Check sheet for the drawn part. Datum: minimum x, y, z corner. Units: mm. A direction names the side the tool comes from. Coordinates: 2 decimals unless noted, no trailing zeros. Order: outer loops, then holes, each group sorted by start corner. A loop starts at its lowest first (then second) coordinate and runs counter-clockwise, first axis right, second up. Notation, with made-up numbers: (-1.5, 58) - (35.5, 58) arc R22 cw to (35.5, 95) - close; hole circle Ø1 at (47, 48). An arc over 180 degrees is marked (long way). One line per item, written item: value. Start each with the question number.
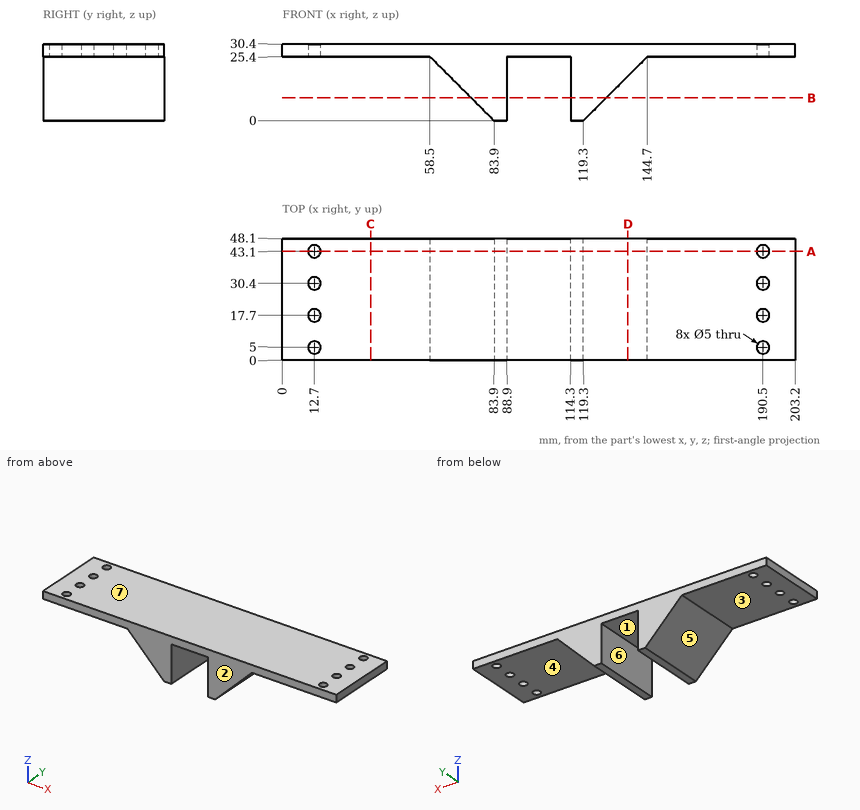
Q1. Material ranges on probe 1 along Y at (x, z) = (190.5, 28.85); probe 2 along X at (y, z) = (17, 27); probe 3 along Y at (x, z) = (190, 29), recorded low to high.
Q2. Cross-section at C-C, the plane x = 35. Enter the section's corners in (y, z).
Q3. Cross-section at B-B, the plane z = 9. Enter the section's corners in (x, y).
Q4. Set-up check for the marked faces 1, 2, 3 and 4: record each of +Z, -Z, +X, -X, +Y, -Y from which the full face is reachable in a straight line by a thin tool's end or side.
Q5. Release check for a two-part mould opening along X. For the marked faces 5, 6 and 7 record: released by +X, released by -X, zero draft, split by the parting line, or undercut.
Q6. Cross-section at A-A, the plane y = 43.1. Count the separate pieces of the cut face and the enclosed holes in it.
Q7. Gauge pin test, flat ends, axial feed: P1, Ø8, axis at y = 38, z = 19, coming from the +X side; P2, Ø6, axis at x = 190.5, y = 5, coming from the -Z side; P3, Ø3, axis at y = 33, z = 7, coming from the +X side. Record the tip position at first contact, or that the pin passes through.
Q8. Cross-section at D-D, the plane x = 137. Enter the section's corners in (y, z), and give its area (3 significant figures).
Check result:
1. probe 1: y = 0 to 2.5, 7.5 to 15.2, 20.2 to 27.9, 32.9 to 40.6, 45.6 to 48.1
1. probe 2: x = 0 to 10.3, 15.1 to 188.1, 192.9 to 203.2
1. probe 3: y = 0 to 2.55, 7.45 to 15.25, 20.15 to 27.95, 32.85 to 40.65, 45.55 to 48.1
2. outline: (0, 25.4) - (48.1, 25.4) - (48.1, 30.4) - (0, 30.4) - close
3. outline: (74.9, 0) - (88.9, 0) - (88.9, 48.1) - (74.9, 48.1) - close; (114.3, 0) - (128.3, 0) - (128.3, 48.1) - (114.3, 48.1) - close
4. face 1: -Z, +Y, -Y
4. face 2: +Z, -Z, +X, -X, -Y
4. face 3: -Z, -X, +Y, -Y
4. face 4: -Z, +X, +Y, -Y
5. face 5: released by -X
5. face 6: undercut
5. face 7: zero draft
6. separate pieces: 3
6. enclosed holes: 0
7. P1: stops at x = 142.3
7. P2: stops at z = 25.4
7. P3: stops at x = 127.8
8. outline: (0, 17.7) - (48.1, 17.7) - (48.1, 30.4) - (0, 30.4) - close
8. area: 611 mm2
